Here's how the part is built. I have some questions about the finished solid (model axes, mm). Round coordinates to 2 decimals unless told otherwise and drop trailing zeros. Write each loop counter-clockwise with the first axis right and the second up, starting at its lowest first coordinate (ties: lowest second). Pieces come first, ordered by that corner, then holes. Notation, with made-up numbers: M -25.75,88 L 23.25,88 A12 ccw 23.25,92 Z; hole C -16.5,61.5 d8. An arc over 180 degrees is marked long. Write item = value, one per line. Start each with the question number.
(1) Will this pin go through, and if not, where does the flat tip stop? pin 1 Ø1.5 at (x, y) = (1, -4) entering from +Z.
(2) I want a section at A-A (z = 10). List the corners of the cut face in (x, y) for me, and give its area (3 significant figures).
(3) I want a section at D-D (x = -4.25). List the corners of the cut face in (y, z) for me, and give its area (3 significant figures).
(4) I need wall thicknesses on line 1 along Z through (x, y) = (0, -1.45); line 2 along X through (y, z) = (-2, -50); line 3 along Z through (x, y) = (1, -2.45). Which ranges of each line are inside material? Lowest first, please.
(5) I want a section at C-C (y = -1.4). List the corners of the cut face in (x, z) for me, and give its area (3 significant figures).
(6) I want a section at B-B (x = 0). List the corners of the cut face in (y, z) for me, and give its area (3 significant figures).
```python
from build123d import *

# Parameters (mm, degrees)
F1_DEPTH = 5
F2_R     = 2.5
F3_DEPTH = 5.001


with BuildPart() as f1:
    # F0 (on Front) → F1 (new body)
    with BuildSketch(Plane.XZ):
        with BuildLine():
            Line((7.5, -50), (7.5, 50))
            Line((7.5, 50), (2.5, 50))
            ThreePointArc((2.5, 50), (0, 47.5), (-2.5, 50))
            Line((-2.5, 50), (-7.5, 50))
            Line((-7.5, 50), (-7.5, -50))
            Line((-7.5, -50), (-2.5, -50))
            ThreePointArc((-2.5, -50), (0, -47.5), (2.5, -50))
            Line((2.5, -50), (7.5, -50))
        make_face()
        with BuildLine():
            Line((2.5, 50), (7.5, 50))
            ThreePointArc((7.5, 50), (0, 57.5), (-7.5, 50))
            Line((-7.5, 50), (-2.5, 50))
            ThreePointArc((-2.5, 50), (0, 52.5), (2.5, 50))
        make_face()
        with BuildLine():
            ThreePointArc((-7.5, -50), (0, -57.5), (7.5, -50))
            Line((7.5, -50), (2.5, -50))
            ThreePointArc((2.5, -50), (0, -52.5), (-2.5, -50))
            Line((-2.5, -50), (-7.5, -50))
        make_face()
    extrude(amount=F1_DEPTH)

    # F2 (on face) → F3 (cut, through all)
    with BuildSketch(Plane.XZ.offset(5)):
        with Locations((0, 10)):
            Circle(F2_R)
    extrude(amount=-F3_DEPTH, mode=Mode.SUBTRACT)


solid = f1.part
```
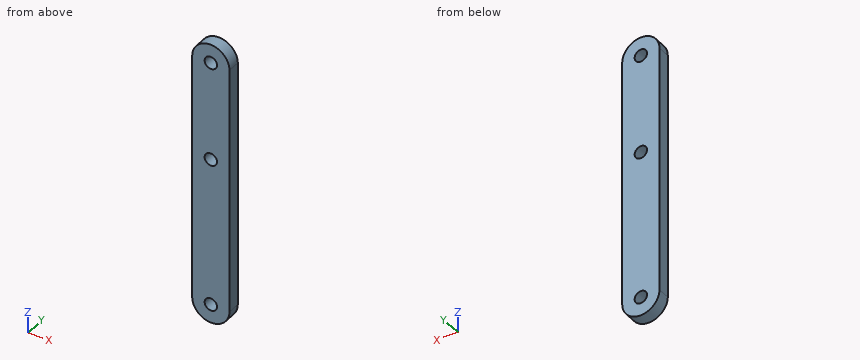
Returned:
q1.pin_1 = 57.5
q2.outline = M -7.5,-5 L -2.5,-5 L -2.5,0 L -7.5,0 Z; M 2.5,-5 L 7.5,-5 L 7.5,0 L 2.5,0 Z
q2.area = 50.0 mm²
q3.outline = M -5,-56.18 L 0,-56.18 L 0,56.18 L -5,56.18 Z
q3.area = 562 mm²
q4.line_1 = -57.5 to -52.5, -47.5 to 7.5, 12.5 to 47.5, 52.5 to 57.5
q4.line_2 = -7.5 to -2.5, 2.5 to 7.5
q4.line_3 = -57.43 to -52.29, -47.71 to 7.71, 12.29 to 47.71, 52.29 to 57.43
q5.outline = M -7.5,-50 A7.5 ccw 7.5,-50 L 7.5,50 A7.5 ccw -7.5,50 Z; hole C 0,-50 d5; hole C 0,10 d5; hole C 0,50 d5
q5.area = 1,620 mm²
q6.outline = M -5,-57.5 L 0,-57.5 L 0,-52.5 L -5,-52.5 Z; M -5,-47.5 L 0,-47.5 L 0,7.5 L -5,7.5 Z; M -5,12.5 L 0,12.5 L 0,47.5 L -5,47.5 Z; M -5,52.5 L 0,52.5 L 0,57.5 L -5,57.5 Z
q6.area = 500 mm²
